Can you work these out from the model? Positions are in its coordinate system, mm. A direction names the side the tool comes from. Give positions to 0.01 mm unless a question says otherwise; leave off trailing zeros. Order: outer loops, then holes, each group sorted by start corner. A loop starts at its lowest first (then second) coordinate and runs counter-clockwise, first axis right, second up. Notation, with made-up numbers: (27.5, 37.25) - (78.5, 37.25) arc R23 ccw to (78.5, 52.25) - close; hole circle Ø1 at (-13, -2.75). An arc over 180 degrees is marked (long way). Answer as a JSON object with one key per item and string values.
```python
from build123d import *

# Parameters (mm, degrees)
SKETCH1_R                 = 41.275
BOSS_EXTRUDE1_DEPTH       = 6.35
FILLET1_R                 = 1.27
F_6_CLEARANCE_HOLE1_D     = 3.7973
F_6_CLEARANCE_HOLE1_DEPTH = 25.4
F_6_CLEARANCE_HOLE1_TIP   = 1.140824014


with BuildPart() as part:
    # Sketch1 → Boss-Extrude1 (new body)
    with BuildSketch(Plane.XY):
        with BuildLine():
            Line((-23.736177688, -34.925), (-57.15, -34.925))
            Line((-57.15, -34.925), (-57.15, -47.625))
            Line((-57.15, -47.625), (57.15, -47.625))
            Line((57.15, -47.625), (57.15, -34.925))
            Line((57.15, -34.925), (23.736177688, -34.925))
            ThreePointArc((23.736177688, -34.925), (0, 42.2275), (-23.736177688, -34.925))
        make_face()
        Circle(SKETCH1_R, mode=Mode.SUBTRACT)
    extrude(amount=BOSS_EXTRUDE1_DEPTH)

    # Fillet1
    fillet1_edges = [part.edges().sort_by_distance(p)[0] for p in [
        (-23.736177688, -34.925, 3.175),
        (23.736177688, -34.925, 3.175),
    ]]
    fillet(fillet1_edges, radius=FILLET1_R)

    # #6 Clearance Hole1
    with Locations(Plane.XZ.offset(47.625)):
        with Locations((-52.3875, 3.175), (52.3875, 3.175)):
            Hole(F_6_CLEARANCE_HOLE1_D / 2, depth=F_6_CLEARANCE_HOLE1_DEPTH)
            with Locations((0, 0, -(F_6_CLEARANCE_HOLE1_DEPTH + F_6_CLEARANCE_HOLE1_TIP / 2))):  # 118° drill point
                Cone(0, F_6_CLEARANCE_HOLE1_D / 2, F_6_CLEARANCE_HOLE1_TIP, mode=Mode.SUBTRACT)


solid = part.part
```
Q1. I'm going to push flat-ended pins straight in: pin 1 Ø3 at (y, z) = (-4.5, 5) entering from -X; pin 2 Ø3 at (x, z) = (49, 4) entering from +Y (3 decimals); pin 3 Ø2 at (x, z) = (-23, 2) entering from +Y. Where does each tip first touch, or does it pass through?
Recorded:
{"pin 1": "stops at x = -42.12", "pin 2": "stops at y = -34.925", "pin 3": "stops at y = 36.04"}
Q2. We'd pull the mould along X, two halves only. Please class faces 1 (the face through (-57.15, -41, 3)), 2 (the face through (-8.948, -40.293, 3.131)), 3 (the face through (43, -34.925, 3)): released by +X, released by -X, zero draft, split by the parting line, or undercut.
Recorded:
{"face 1": "released by -X", "face 2": "undercut", "face 3": "zero draft"}
Q3. If we section it at C-C, the plane x = 32.5: Please give me the cut outline in (y, z) (3 decimals), then the cut area to 3 significant figures.
Recorded:
{"outline": "(-47.625, 0) - (-34.925, 0) - (-34.925, 6.35) - (-47.625, 6.35) - close; (-26.961, 0) - (-25.444, 0) - (-25.444, 6.35) - (-26.961, 6.35) - close; (25.444, 0) - (26.961, 0) - (26.961, 6.35) - (25.444, 6.35) - close", "area": "99.9 mm^2"}
Q4. If we section it at D-D, the plane x = -36.5: Please give me the cut outline in (y, z) (3 decimals), then the cut area to 3 significant figures.
Recorded:
{"outline": "(-47.625, 0) - (-34.925, 0) - (-34.925, 6.35) - (-47.625, 6.35) - close; (-21.235, 0) - (-19.271, 0) - (-19.271, 6.35) - (-21.235, 6.35) - close; (19.271, 0) - (21.235, 0) - (21.235, 6.35) - (19.271, 6.35) - close", "area": "106 mm^2"}
Q5. Which directions (+Z, -Z, +X, -X, +Y, -Y) give clear straight access to the entire face, cutting with the end or side of a thin tool? Please do faces 4 (the face through (-42, -34.925, 3)), 5 (the face through (57.15, -41, 3)).
Recorded:
{"face 4": "+Z, -Z, -X", "face 5": "+Z, -Z, +X, +Y, -Y"}
Q6. I need wall thicknesses on L1, parallel to X at y = -35, z = 1.75; L2, parallel to Y at x = -34, z = 1 (3 decimals); L3, parallel to Y at x = -32.5, z = 1.75 (3 decimals). Which ranges of each line are inside material? Lowest first, please.
Recorded:
{"L1": "x = -57.15 to -53.64, -51.13 to -21.88, 21.88 to 51.13, 53.64 to 57.15", "L2": "y = -47.625 to -34.925, -25.043 to -23.401, 23.401 to 25.043", "L3": "y = -47.625 to -34.925, -26.961 to -25.444, 25.444 to 26.961"}
